from build123d import *

# Parameters (mm, degrees)
F1_DEPTH = 63.5
F0_W     = 25.4
F0_H     = 19.05
F2_DEPTH = 25.4
F3_DEPTH = 7.9375


with BuildPart() as f1:
    # F0 (on Front) → F1 (new body, symmetric)
    with BuildSketch(Plane.XZ):
        Polygon((-41.275, -9.525), (41.275, -9.525), (41.275, 9.525), (22.225, 9.525), (-41.275, 9.525), align=None)
    extrude(amount=F1_DEPTH, both=True)

    # F0 (on Front) → F2 (join, symmetric)
    with BuildSketch(Plane.XZ):
        with BuildLine():
            Line((22.225, 9.525), (41.275, 9.525))
            Line((41.275, 9.525), (41.275, 27.0002))
            ThreePointArc((41.275, 27.0002), (45.9246798487, 38.2255201513), (57.15, 42.8752))
            Line((57.15, 42.8752), (60.325, 42.8752))
            Line((60.325, 42.8752), (60.325, 61.9252))
            Line((60.325, 61.9252), (57.15, 61.9252))
            add(Edge.make_bspline(
                [(56.4347952679, 61.9178761425), (56.6731549008, 61.920563236), (56.9115579755, 61.9230028803), (57.15, 61.9252)],
                knots=[110.8800193366, 110.8800193366, 110.8800193366, 110.8800193366, 111.5045361635, 111.5045361635, 111.5045361635, 111.5045361635], degree=3))
            ThreePointArc((56.4347952679, 61.9178761425), (32.2027140728, 51.4417332961), (22.225, 27.0002))
            Line((22.225, 27.0002), (22.225, 9.525))
        make_face()
        with Locations((73.025, 52.4002)):
            Rectangle(F0_W, F0_H)
    extrude(amount=F2_DEPTH, both=True)

    # F0 (on Front) → F3 (join, symmetric)
    with BuildSketch(Plane.XZ):
        with BuildLine():
            add(Edge.make_bspline(
                [(-41.275, 9.525), (-26.8350750497, 53.1635386099), (14.1151658157, 61.4407953484), (56.4347952679, 61.9178761425)],
                knots=[0, 0, 0, 0, 110.8800193366, 110.8800193366, 110.8800193366, 110.8800193366], degree=3))
            Line((-41.275, 9.525), (22.225, 9.525))
            Line((22.225, 9.525), (22.225, 27.0002))
            ThreePointArc((22.225, 27.0002), (32.2027140728, 51.4417332961), (56.4347952679, 61.9178761425))
        make_face()
    extrude(amount=F3_DEPTH, both=True)

    # F0 (on Front) → F4 (revolve)
    with BuildSketch(Plane.XZ):
        Polygon((85.725, 61.9252), (85.725, 42.8752), (85.725, 38.1), (111.125, 38.1), (111.125, 66.675), (85.725, 66.675), align=None)
    revolve(axis=Axis((85.725, 0, 52.3875), (0, 0, -1)))


solid = f1.part
Read the model definition and answer for the solid it produces. Units are mm, in the model's axes. A direction names the side the tool comes from. Coordinates: 2 decimals unless noted, no trailing zeros. Write each loop counter-clockwise with the first axis right and the second up, starting at its lowest first coordinate (ties: lowest second). Pieces come first, ordered by that corner, then holes. Notation, with made-up numbers: (35, 51) - (67, 51) arc R22 cw to (67, 83) - close; hole circle Ø9 at (63, 65). An arc over 180 degrees is marked (long way). One line per question, with ' | ' between items.
Q1. For faces 1 (the cylindrical face through (45.8, -0.4, 38.1)), 2 (the flat face through (46, -25.4, 42)), 3 (the flat face through (22.225, -17, 18)), 4 (the flat face through (46, 25.4, 42)), determine the directions among +Z, -Z, +X, -X, +Y, -Y from which every point of the face is accessible in a straight line to the end or side of a thin tool.
Result set:
face 1: -Z, +Y, -Y | face 2: +Z, +X, -X, -Y | face 3: +Z, -X, -Y | face 4: +Z, +X, -X, +Y
Q2. Find section A-A, the plane x = 84. Write down the section's boundary in (y, z) (3 decimals).
Result set:
outline: (-25.4, 42.875) - (-25.341, 42.875) - (-25.341, 38.1) - (25.341, 38.1) - (25.341, 42.875) - (25.4, 42.875) - (25.4, 61.925) - (25.341, 61.925) - (25.341, 66.675) - (-25.341, 66.675) - (-25.341, 61.925) - (-25.4, 61.925) - close
Q3. Each of these flat-tipped pins is pushed along its axis until it touches: P1, Ø8, axis at y = 16, z = 23.5, coming from the +X side; P2, Ø23, axis at x = 78, y = 3, coming from the -Z side; P3, Ø1.5, axis at x = 37.5, y = 9.5, coming from the +Z side. Where does it stop, or does it pass through?
Result set:
P1: x = 41.28 | P2: z = 38.1 | P3: z = 56.37
Q4. Consider L1, parallel to X at y = 50, z = -6 (3 decimals); L2, parallel to Y at x = 22.5, z = 12; L3, parallel to Z at x = 82.5, y = 9 (3 decimals). Determine where each line is inside the solid, lowest interval first. Write a range as [from, to].
Result set:
L1: [-41.275, 41.275] | L2: [-25.4, 25.4] | L3: [38.1, 66.675]
Q5. Find section B-B, the plane y = -35.5. Write down the section's boundary in (x, z) (3 decimals).
Result set:
outline: (-41.275, -9.525) - (41.275, -9.525) - (41.275, 9.525) - (-41.275, 9.525) - close
